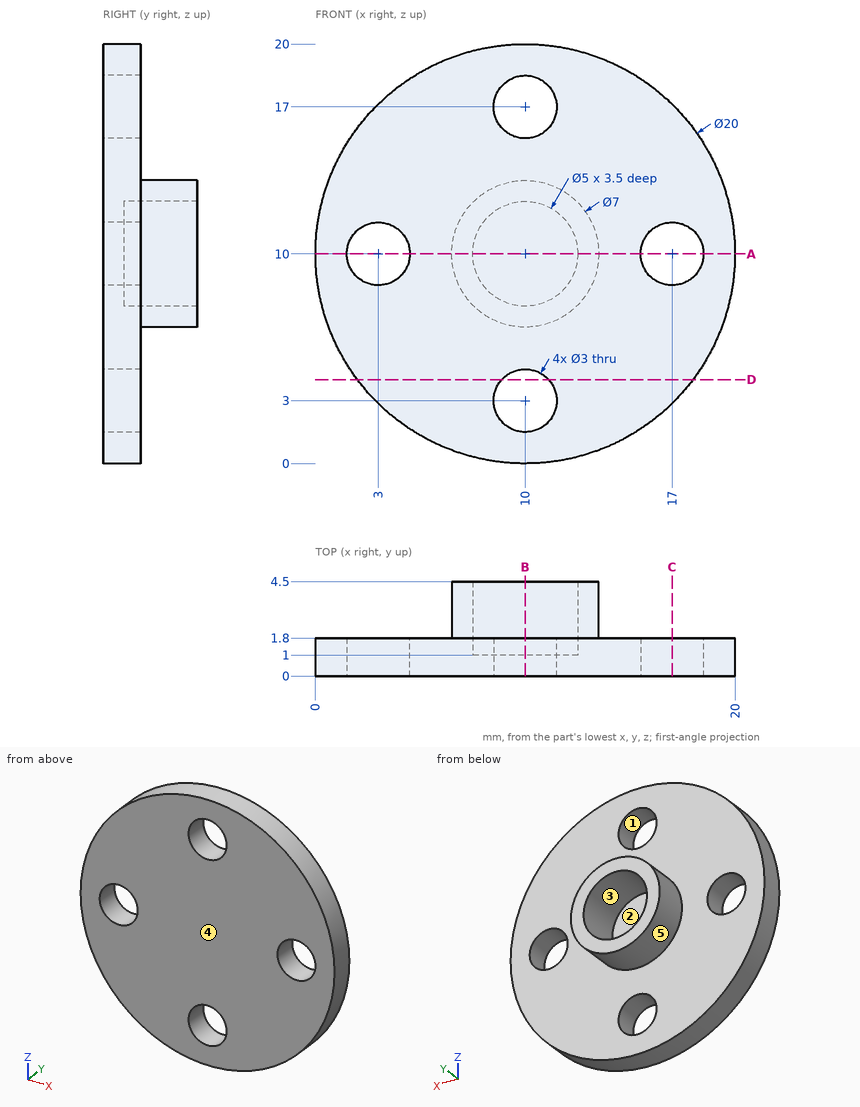
Geometry: see drawing. Coordinates: mm, zero at the bounding-box minimum. A direction names the side the tool comes from. Give positions to 0.01 mm unless a question says otherwise; leave off trailing zeros. Order: outer loops, then holes, each group sorted by start corner. A loop starts at its lowest first (then second) coordinate and runs counter-clockwise, first axis right, second up. Notation, with made-up numbers: (29, -25) - (37, -25) arc R23 cw to (37, -1) - close; hole circle Ø9 at (68, 5.25). An arc over 180 degrees is marked (long way). One line per item, written item: value.
1. Cut plane C-C, the plane x = 17. Output: boundary loops of the cut face in (y, z), and give its area (3 significant figures).
Determined:
outline: (0, 2.86) - (1.8, 2.86) - (1.8, 8.5) - (0, 8.5) - close; (0, 11.5) - (1.8, 11.5) - (1.8, 17.14) - (0, 17.14) - close
area: 20.3 mm2
2. Draft query along Z for the marked faces 3, 4 and 5. Return one class per face: released by +Z, released by -Z, zero draft, split by the parting line, or undercut.
Determined:
face 3: undercut
face 4: zero draft
face 5: split by the parting line
3. Cut plane D-D, the plane z = 4. Output: boundary loops of the cut face in (x, y), and give its area (3 significant figures).
Determined:
outline: (2, 0) - (8.88, 0) - (8.88, 1.8) - (2, 1.8) - close; (11.12, 0) - (18, 0) - (18, 1.8) - (11.12, 1.8) - close
area: 24.8 mm2
4. Line query: probe 1 along Z at (x, y) = (10, 0.4); probe 2 along Z at (x, y) = (10, 1.3); probe 3 along X at (y, z) = (1.6, 10.5). Output: solid intervals per line, ascending.
Determined:
probe 1: 0 to 1.5, 4.5 to 15.5, 18.5 to 20
probe 2: 0 to 1.5, 4.5 to 7.5, 12.5 to 15.5, 18.5 to 20
probe 3: 0.01 to 1.59, 4.41 to 7.55, 12.45 to 15.59, 18.41 to 19.99
5. Reachability of the marked faces 1 and 2 from +Z, -Z, +X, -X, +Y, -Y: full face, straight path, thin tool, end or side. Return the list, or none.
Determined:
face 1: +Y, -Y
face 2: +Y
6. Cut plane B-B, the plane x = 10. Output: boundary loops of the cut face in (y, z).
Determined:
outline: (0, 0) - (1.8, 0) - (1.8, 1.5) - (0, 1.5) - close; (0, 4.5) - (1.8, 4.5) - (1.8, 6.5) - (4.5, 6.5) - (4.5, 7.5) - (1, 7.5) - (1, 12.5) - (4.5, 12.5) - (4.5, 13.5) - (1.8, 13.5) - (1.8, 15.5) - (0, 15.5) - close; (0, 18.5) - (1.8, 18.5) - (1.8, 20) - (0, 20) - close
7. Cut plane A-A, the plane z = 10. Output: boundary loops of the cut face in (x, y).
Determined:
outline: (0, 0) - (1.5, 0) - (1.5, 1.8) - (0, 1.8) - close; (4.5, 0) - (15.5, 0) - (15.5, 1.8) - (13.5, 1.8) - (13.5, 4.5) - (12.5, 4.5) - (12.5, 1) - (7.5, 1) - (7.5, 4.5) - (6.5, 4.5) - (6.5, 1.8) - (4.5, 1.8) - close; (18.5, 0) - (20, 0) - (20, 1.8) - (18.5, 1.8) - close
8. Pin query (flat end, axial travel): pin 1 Ø2.5 at (x, z) = (17, 10) entering from +Y; pin 2 Ø4 at (x, z) = (10, 10) entering from +Y; pin 3 Ø1 at (y, z) = (2, 2.5) entering from +X; pin 4 Ø2 at (y, z) = (1.5, 16) entering from -X. Return the tip coordinate at first contact, or that it passes through.
Determined:
pin 1: through
pin 2: y = 1
pin 3: x = 17.1
pin 4: x = 1.34
